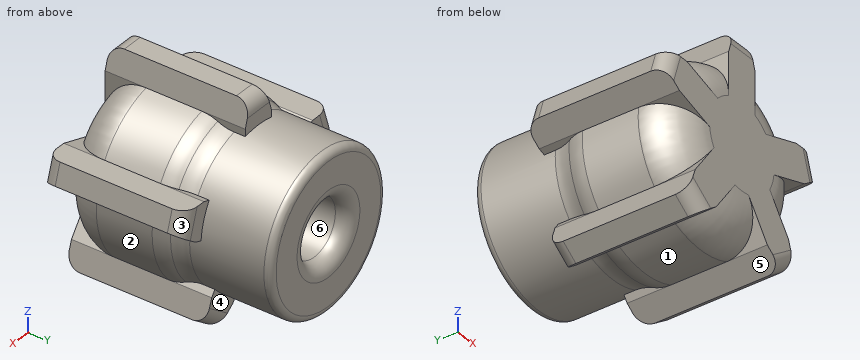
from build123d import *

# Parameters (mm, degrees)
SKETCH3_R           = 4
CUT_EXTRUDE2_DEPTH  = 29
FILLET2_R           = 2
BOSS_EXTRUDE1_DEPTH = 20
FILLET3_R           = 2


with BuildPart() as part:
    # Sketch1 → Revolve1 (revolve)
    with BuildSketch(Plane.XY):
        with BuildLine():
            Line((0, 30), (0, 0))
            Line((0, 0), (-6.164929537, 0))
            ThreePointArc((-6.164929537, 0), (-10.29094743, 1.70905257), (-12, 5.835070463))
            Line((-12, 5.835070463), (-12, 13.798025689))
            ThreePointArc((-12, 13.798025689), (-11.875902596, 14.955923247), (-11.50924738, 16.061224505))
            ThreePointArc((-11.50924738, 16.061224505), (-11.128774204, 17.208180724), (-11, 18.409715414))
            Line((-11, 18.409715414), (-11, 29))
            ThreePointArc((-11, 29), (-10.707106781, 29.707106781), (-10, 30))
            Line((-10, 30), (0, 30))
        make_face()
    revolve(axis=Axis((0, 30, 0), (0, -1, 0)))

    # Sketch3 → Cut-Extrude2 (cut)
    with BuildSketch(Plane(origin=(0, 30, 0), x_dir=(1, 0, 0), z_dir=(0, 1, 0))):
        Circle(SKETCH3_R)
    extrude(amount=-CUT_EXTRUDE2_DEPTH, mode=Mode.SUBTRACT)

    # Fillet2
    fillet2_edges = [part.edges().sort_by_distance(p)[0] for p in [
        (-4, 30, 0),
    ]]
    fillet(fillet2_edges, radius=FILLET2_R)

    # Sketch2 → Boss-Extrude1 (add)
    with BuildSketch(Plane.XZ):
        Polygon((-1.5, 15), (1.5, 15), (2.5, 11.736694594), (2.5, 5.635277828), (-2.5, 5.635277828), (-2.5, 11.736694594), align=None)
        Polygon((10.389717388, 6.004479378), (4.586925213, 4.119037908), (6.132010185, -0.636244674), (11.93480236, 1.249196797), (14.729373236, 3.208670141), (13.802322253, 6.06183969), align=None)
        Polygon((8.921198479, -8.025722254), (5.334875686, -3.0895724), (1.289790714, -6.028498661), (4.876113507, -10.964648515), (7.603253293, -13.016932794), (10.030304276, -11.253577037), align=None)
        Polygon((-4.876113507, -10.964648515), (-1.289790714, -6.028498661), (-5.334875686, -3.0895724), (-8.921198479, -8.025722254), (-10.030304276, -11.253577037), (-7.603253293, -13.016932794), align=None)
        Polygon((-11.93480236, 1.249196797), (-6.132010185, -0.636244674), (-4.586925213, 4.119037908), (-10.389717388, 6.004479378), (-13.802322253, 6.06183969), (-14.729373236, 3.208670141), align=None)
    extrude(amount=-BOSS_EXTRUDE1_DEPTH)

    # Fillet3
    fillet3_edges = [part.edges().sort_by_distance(p)[0] for p in [
        (-8.816778784, 20, -12.135254916),
        (-8.816778784, 0, -12.135254916),
        (-14.265847744, 20, 4.635254916),
        (-14.265847744, 0, 4.635254916),
        (0, 20, 15),
        (0, 0, 15),
        (14.265847744, 20, 4.635254916),
        (14.265847744, 0, 4.635254916),
        (8.816778784, 20, -12.135254916),
        (8.816778784, 0, -12.135254916),
    ]]
    fillet(fillet3_edges, radius=FILLET3_R)


solid = part.part
Geometry: final body of the model. Coordinates: model frame, mm. Face numbers are marked on the shaded views. A direction names the side the tool comes from. Round coordinates to 2 decimals unless told otherwise and drop trailing zeros. Loops run counter-clockwise (first coordinate to the right, second up) from the corner with the lowest first, then second, coordinate; pieces in that order, holes last. Notation, with made-up numbers: (11, 33) - (21, 33) arc R17 cw to (21, 50) - close; hole circle Ø2 at (-39.5, -24.5). An arc over 180 degrees is marked (long way). Write each question's results on one line, items separated by ' | '. Start each with the question number.
1) Access query for the marked faces 4, 5 and 6. Directions: +Z, -Z, +X, -X, +Y, -Y. A direction counts if a zero-diameter tool reaches every point of the face in a straight line with its end or side. Return the directions, or none.
2) Line query: probe 1 along X at (y, z) = (21.75, 0); probe 2 along Z at (x, y) = (0, 11.25); probe 3 along Y at (x, z) = (-0.25, 13). Output: solid intervals per line, ascending. Write a range as [from, to].
3) Cut plane C-C on z = 0. Return loops of the section in (x, y), then the cut area to 3 significant figures.
4) Cut plane A-A on y = 7. Return loops of the section in (x, z).
5) Cut plane B-B on x = 0. Return loops of the section in (y, z).
6) Cut plane D-D on y = 26. Return loops of the section in (x, z), then the cut area to 3 significant figures.
7) Mould query, pull axis Z, two halves, no side actions, for the marked faces 1, 2 and 3. Classes: released by +Z, released by -Z, zero draft, split by the parting line, or undercut.
8) First-contact query: P1, Ø0.7, axis at x = 1, z = 12.5, coming from the +Y side; P2, Ø5, axis at x = -5.5, y = 15, coming from the +Z side; P3, Ø6, axis at y = 20, z = -3.5, coming from the +X side. Flat tips, straight axial feed; report the tip coordinate or a pass-through.
Verdict:
1) face 4: -Z, +X, +Y | face 5: -Z, +Y, -Y | face 6: +Y
2) probe 1: x = [-11, -4], [4, 11] | probe 2: z = [-12, -4], [4, 15] | probe 3: y = [0, 20]
3) outline: (-12, 5.84) arc R5.84 ccw to (-8.09, 0.33) - (-8.09, 0) - (8.09, 0) - (8.09, 0.33) arc R5.84 ccw to (12, 5.84) - (12, 13.8) arc R5.46 ccw to (11.51, 16.06) arc R5.67 cw to (11, 18.41) - (11, 29) arc R1 ccw to (10, 30) - (6, 30) arc R2 ccw to (4, 28) - (4, 1) - (-4, 1) - (-4, 28) arc R2 ccw to (-6, 30) - (-10, 30) arc R1 ccw to (-11, 29) - (-11, 18.41) arc R5.67 cw to (-11.51, 16.06) arc R5.46 ccw to (-12, 13.8) - close | area: 444 mm2
4) outline: (-14.73, 3.21) - (-11.93, 1.25) arc R12 ccw to (-8.92, -8.03) - (-10.03, -11.25) - (-7.6, -13.02) - (-4.88, -10.96) arc R12 ccw to (4.88, -10.96) - (7.6, -13.02) - (10.03, -11.25) - (8.92, -8.03) arc R12 ccw to (11.93, 1.25) - (14.73, 3.21) - (13.8, 6.06) - (10.39, 6) arc R12 ccw to (2.5, 11.74) - (1.5, 15) - (-1.5, 15) - (-2.5, 11.74) arc R12 ccw to (-10.39, 6) - (-13.8, 6.06) - close; hole circle Ø8 at (0, 0)
5) outline: (0, -6.16) arc R5.84 ccw to (5.84, -12) - (13.8, -12) arc R5.46 ccw to (16.06, -11.51) arc R5.67 cw to (18.41, -11) - (29, -11) arc R1 ccw to (30, -10) - (30, -6) arc R2 ccw to (28, -4) - (1, -4) - (1, 4) - (28, 4) arc R2 ccw to (30, 6) - (30, 10) arc R1 ccw to (29, 11) - (20, 11) - (20, 13) arc R2 ccw to (18, 15) - (2, 15) arc R2 ccw to (0, 13) - close
6) outline: circle Ø22 at (0, 0); hole circle Ø8 at (0, 0) | area: 330 mm2
7) face 1: released by -Z | face 2: undercut | face 3: released by +Z
8) P1: stops at y = 20 | P2: stops at z = 11.57 | P3: stops at x = 10.99
